Read the model definition and answer for the solid it produces. Units are mm, in the model's axes. A direction names the side the tool comes from. Coordinates: 2 decimals unless noted, no trailing zeros. Write each loop counter-clockwise with the first axis right and the second up, starting at its lowest first coordinate (ties: lowest second). Pieces come first, ordered by that corner, then holes. Notation, with made-up numbers: (-20, 27.25) -> (-4, 27.25) arc R21 ccw to (-4, 45.25) -> close; hole circle Ø11 at (11, -17). An arc over 180 degrees is marked (long way). One line per item, written item: value. Start each with the question number.
1. Given P1, Ø2, axis at x = -24.5, z = 11, coming from the -Y side; P2, Ø2, axis at x = 23, y = 6, coming from the +Z side; P3, Ø1, axis at y = 1, z = 11, coming from the -X side, each flat-ended and moving along its own axis, determine where each tip first touches the part or whether it passes through.
2. Find section C-C, the plane z = 7.75. Write down the section's boundary in (x, y).
3. Consider line 1 along Y through (x, z) = (28, 1.2); line 2 along X through (y, z) = (-1.75, 1.5); line 3 along X through (y, z) = (0, 7.5). Determine where each line is inside the solid, lowest interval first.
4. For faces 1 (the flat face through (9, 0, 3)), 2 (the flat face through (1, 0, 1)), 3 (the flat face through (-28, 0, 10)), determine the directions among +Z, -Z, +X, -X, +Y, -Y from which every point of the face is accessible in a straight line to the end or side of a thin tool.
5. Find section B-B, the plane x = -21. Write down the section's boundary in (y, z), and give its area (3 significant figures).
6. Find section A-A, the plane y = 2.5. Write down the section's boundary in (x, z), and give its area (3 significant figures).
7. Find section D-D, the plane x = 20. Write down the section's boundary in (y, z), and give its area (3 significant figures).
8. For a pull along X with two mould halves and no side action, classify faces 4 (the cylindrical face through (26.69, 4.25, 1.48)), 5 (the flat face through (-13, 0, 6)), 6 (the flat face through (-16, 0, 10)) as pulls with the +X half, pulls with the -X half, needs draft (parallel to the pull), parting line crosses it, or undercut.
```python
from build123d import *

# Parameters (mm, degrees)
SKETCH050_W     = 62
SKETCH050_H     = 16.5
SKETCH050_R     = 1.65
SKETCH050_W_2   = 13
SKETCH050_H_2   = 3.2
SKETCH050_W_3   = 4
SKETCH050_H_3   = 10.9
PAD010_DEPTH    = 3
SKETCH051_W     = 18
SKETCH051_H     = 16.5
PAD011_DEPTH    = 10
SKETCH052_R     = 1.65
POCKET031_DEPTH = 31.001
SKETCH053_W     = 6
SKETCH053_H     = 16.5
PAD012_DEPTH    = 2
SKETCH054_R     = 1.65
POCKET032_DEPTH = 12.001


with BuildPart() as part:
    # Sketch050 → Pad010 (new body)
    with BuildSketch(Plane.XY):
        Rectangle(SKETCH050_W, SKETCH050_H)
        with Locations((-21, 0)):
            Circle(SKETCH050_R, mode=Mode.SUBTRACT)
        with Locations((28, 5.25)):
            Circle(SKETCH050_R, mode=Mode.SUBTRACT)
        with Locations((9, 5.25)):
            Circle(SKETCH050_R, mode=Mode.SUBTRACT)
        with Locations((18.5, -1.65)):
            Rectangle(SKETCH050_W_2, SKETCH050_H_2, mode=Mode.SUBTRACT)
        with Locations((3, 0)):
            Rectangle(SKETCH050_W_3, SKETCH050_H_3, mode=Mode.SUBTRACT)
    extrude(amount=PAD010_DEPTH)

    # Sketch051 → Pad011 (join)
    with BuildSketch(Plane.XY):
        with Locations((-22, 0)):
            Rectangle(SKETCH051_W, SKETCH051_H)
    extrude(amount=PAD011_DEPTH)

    # Sketch052 → Pocket031 (cut, through all)
    with BuildSketch(Plane.YZ):
        with Locations((0, 13)):
            Circle(SKETCH052_R)
    extrude(amount=-POCKET031_DEPTH, mode=Mode.SUBTRACT)

    # Sketch053 → Pad012 (join)
    with BuildSketch(Plane.XY.offset(10)):
        with Locations((-21, 0)):
            Rectangle(SKETCH053_W, SKETCH053_H)
    extrude(amount=PAD012_DEPTH)

    # Sketch054 → Pocket032 (cut, through all)
    with BuildSketch(Plane.XY):
        with Locations((-21, 0)):
            Circle(SKETCH054_R)
    extrude(amount=POCKET032_DEPTH, mode=Mode.SUBTRACT)


solid = part.part
```
Answer block:
1. P1: stops at y = -8.25
1. P2: stops at z = 3
1. P3: stops at x = -24
2. outline: (-31, -8.25) -> (-13, -8.25) -> (-13, 8.25) -> (-31, 8.25) -> close; hole circle Ø3.3 at (-21, 0)
3. line 1: y = -8.25 to 3.6, 6.9 to 8.25
3. line 2: x = -31 to 1, 5 to 12, 25 to 31
3. line 3: x = -31 to -22.65, -19.35 to -13
4. face 1: +Z, +X, +Y, -Y
4. face 2: +Z, -Z
4. face 3: +Z, -X, +Y, -Y
5. outline: (-8.25, 0) -> (-1.65, 0) -> (-1.65, 12) -> (-8.25, 12) -> close; (1.65, 0) -> (8.25, 0) -> (8.25, 12) -> (1.65, 12) -> close
5. area: 158 mm2
6. outline: (-31, 0) -> (1, 0) -> (1, 3) -> (-13, 3) -> (-13, 10) -> (-18, 10) -> (-18, 12) -> (-24, 12) -> (-24, 10) -> (-31, 10) -> close; (5, 0) -> (31, 0) -> (31, 3) -> (5, 3) -> close
6. area: 312 mm2
7. outline: (-8.25, 0) -> (-3.25, 0) -> (-3.25, 3) -> (-8.25, 3) -> close; (-0.05, 0) -> (8.25, 0) -> (8.25, 3) -> (-0.05, 3) -> close
7. area: 39.9 mm2
8. face 4: undercut
8. face 5: pulls with the +X half
8. face 6: needs draft
